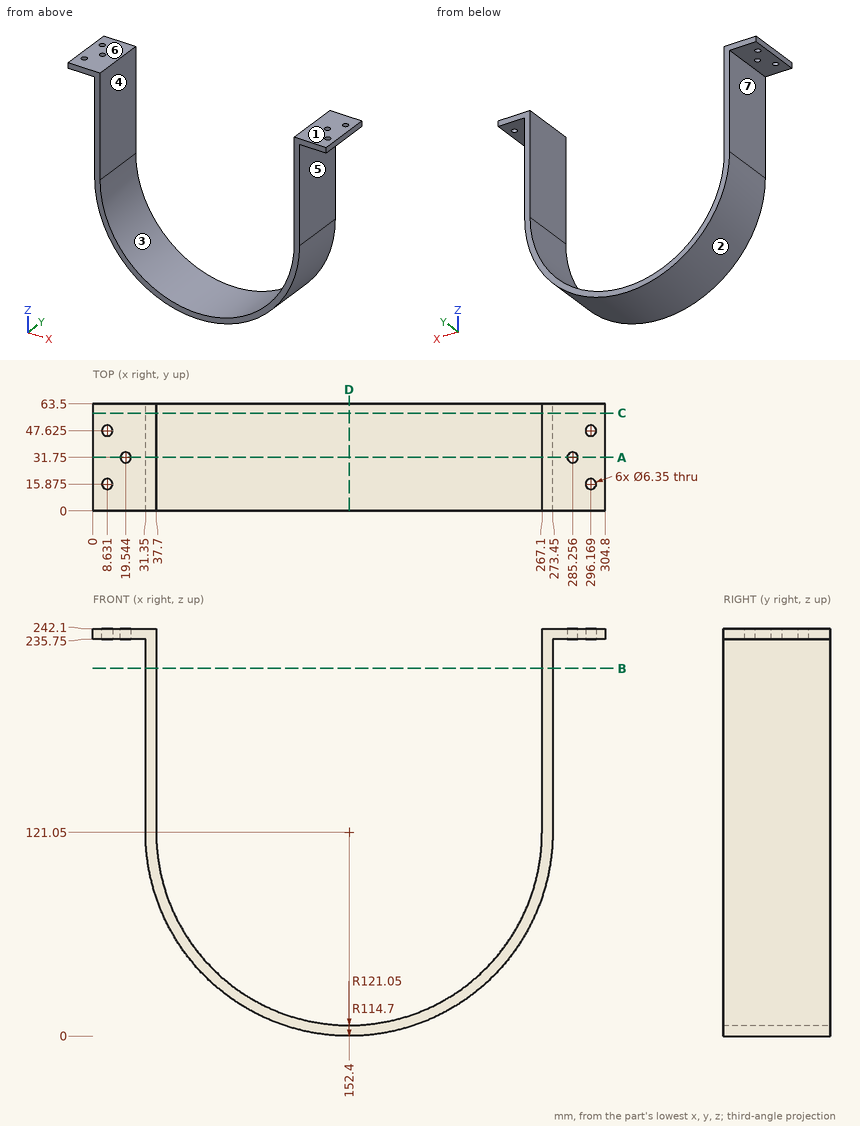
Print and shaded views of the part. All mm, measured from the part's lowest x, y and z. A direction names the side the tool comes from. Round coordinates to 2 decimals unless told otherwise and drop trailing zeros. Write each loop counter-clockwise with the first axis right and the second up, starting at its lowest first coordinate (ties: lowest second). Pieces come first, ordered by that corner, then holes. Notation, with made-up numbers: (86, -22.75) -> (108, -22.75) arc R25 ccw to (108, -9.75) -> close; hole circle Ø4 at (49, -17.5). An arc over 180 degrees is marked (long way). Return JSON: item names as keys, results as strings. Group by question number.
Q1. Mould opens along X. For the marked faces 1, 2 and 3 say: pulls with the +X half, pulls with the -X half, needs draft (parallel to the pull), parting line crosses it, or undercut.
Q2. Saw through at A-A on y = 31.75. Write the cut outline in (x, z).
Q3. Saw through at D-D on x = 152.4. Write the cut outline in (y, z), plus the area to 3 significant figures.
Q4. Saw through at B-B on z = 218.5. Write the cut outline in (x, y).
Q5. Pin check, flat tips, straight feed: pin 1 (10 mm diameter, centred on x = 8.63, y = 47.62, fed in from +Z); pin 2 (5.5 mm diameter, centred on x = 19.54, y = 31.75, fed in from -Z); pin 3 (10 mm diameter, centred on x = 115.5, y = 51, fed in from -Z); pin 4 (8 mm diameter, centred on y = 27.5, z = 186, fed in from -X). Stop position of each tip, or through.
Q6. Saw through at C-C on y = 58. Write the cut outline in (x, z).
Q7. Probe L1, parallel to X at y = 17.5, z = 191; L2, parallel to Z at x = 30.5, y = 23. List the from-to ranges inside material, lowest first. Write a range as [from, to].
Q8. Which spindle directions (+Z, -Z, +X, -X, +Y, -Y) get a long thin tool onto all of the face, cutting with end or side? Do the marked faces 4, 5, 6 and 7. Say none if no direction does.
Answer:
{
 "1": {"face 1": "needs draft", "face 2": "parting line crosses it", "face 3": "undercut"},
 "2": {"outline": "(0, 235.75) -> (16.37, 235.75) -> (16.37, 242.1) -> (0, 242.1) -> close; (22.72, 235.75) -> (31.35, 235.75) -> (31.35, 121.05) arc R121.05 ccw to (273.45, 121.05) -> (273.45, 235.75) -> (282.08, 235.75) -> (282.08, 242.1) -> (267.1, 242.1) -> (267.1, 121.05) arc R114.7 cw to (37.7, 121.05) -> (37.7, 242.1) -> (22.72, 242.1) -> close; (288.43, 235.75) -> (304.8, 235.75) -> (304.8, 242.1) -> (288.43, 242.1) -> close"},
 "3": {"outline": "(0, 0) -> (63.5, 0) -> (63.5, 6.35) -> (0, 6.35) -> close", "area": "403 mm2"},
 "4": {"outline": "(31.35, 0) -> (37.7, 0) -> (37.7, 63.5) -> (31.35, 63.5) -> close; (267.1, 0) -> (273.45, 0) -> (273.45, 63.5) -> (267.1, 63.5) -> close"},
 "5": {"pin 1": "z = 242.1", "pin 2": "through", "pin 3": "z = 4.28", "pin 4": "x = 31.35"},
 "6": {"outline": "(0, 235.75) -> (31.35, 235.75) -> (31.35, 121.05) arc R121.05 ccw to (273.45, 121.05) -> (273.45, 235.75) -> (304.8, 235.75) -> (304.8, 242.1) -> (267.1, 242.1) -> (267.1, 121.05) arc R114.7 cw to (37.7, 121.05) -> (37.7, 242.1) -> (0, 242.1) -> close"},
 "7": {"L1": "[31.35, 37.7], [267.1, 273.45]", "L2": "[235.75, 242.1]"},
 "8": {"face 4": "+Z, +Y, -Y", "face 5": "-Z, +X, +Y, -Y", "face 6": "+Z, +X, -X, +Y, -Y", "face 7": "-Z, -X, +Y, -Y"}
}
